```python
from build123d import *

# Parameters (mm, degrees)
ESQUISSE20_R        = 1.5
BOSS_EXTRU_18_DEPTH = 3


with BuildPart() as part:
    # Esquisse20 → Boss.-Extru.18 (new body)
    with BuildSketch(Plane.XY):
        with BuildLine():
            Line((110.974145272, 39.836071078), (121.886788051, 41.354939341))
            Line((121.886788051, 41.354939341), (126.749523122, 37.68045145))
            Line((126.749523122, 37.68045145), (136.453547574, 39.031099049))
            ThreePointArc((136.453547574, 39.031099049), (136.70394605, 39.25838517), (136.583626314, 39.574425576))
            Line((136.583626314, 39.574425576), (122.215724565, 49.579536305))
            Line((122.215724565, 49.579536305), (109.446142116, 47.334623838))
            ThreePointArc((109.446142116, 47.334623838), (109.157676293, 47.445546281), (109.120229419, 47.752326416))
            ThreePointArc((109.120229419, 47.752326416), (109.228042095, 48.009211598), (109.32429992, 48.270646104))
            ThreePointArc((109.32429992, 48.270646104), (109.335764075, 48.421294196), (109.272350858, 48.558425661))
            ThreePointArc((109.272350858, 48.558425661), (109.097464559, 48.765803687), (108.917279288, 48.968594544))
            ThreePointArc((108.917279288, 48.968594544), (108.79064668, 49.050998774), (108.639910127, 49.061234313))
            ThreePointArc((108.639910127, 49.061234313), (107.261509219, 48.631031321), (106.01862318, 47.895981682))
            ThreePointArc((106.01862318, 47.895981682), (105.838096498, 47.834835241), (105.657168579, 47.894784036))
            ThreePointArc((105.657168579, 47.894784036), (105.512617586, 48.000463717), (105.365584876, 48.10266238))
            ThreePointArc((105.365584876, 48.10266238), (105.21615426, 48.20132177), (105.064410914, 48.296385651))
            ThreePointArc((105.064410914, 48.296385651), (104.94165105, 48.44218958), (104.931503697, 48.632520348))
            ThreePointArc((104.931503697, 48.632520348), (105.15332497, 50.059355658), (105.041782665, 51.499016031))
            ThreePointArc((105.041782665, 51.499016031), (104.976386869, 51.635213184), (104.85290368, 51.722265908))
            ThreePointArc((104.85290368, 51.722265908), (104.597758689, 51.814417397), (104.340318239, 51.899946795))
            ThreePointArc((104.340318239, 51.899946795), (104.189449068, 51.907994647), (104.053789615, 51.841490608))
            ThreePointArc((104.053789615, 51.841490608), (103.075160908, 50.779723434), (102.366314843, 49.521708754))
            ThreePointArc((102.366314843, 49.521708754), (102.240547371, 49.378491042), (102.053884799, 49.339944262))
            ThreePointArc((102.053884799, 49.339944262), (101.875860127, 49.359190054), (101.697426734, 49.374180337))
            ThreePointArc((101.697426734, 49.374180337), (101.518686329, 49.384906567), (101.339740796, 49.39136263))
            ThreePointArc((101.339740796, 49.39136263), (101.160525671, 49.456252605), (101.056572421, 49.616010208))
            ThreePointArc((101.056572421, 49.616010208), (100.535257624, 50.96259647), (99.718828968, 52.153607774))
            ThreePointArc((99.718828968, 52.153607774), (99.59409597, 52.23886007), (99.44363003, 52.252508346))
            ThreePointArc((99.44363003, 52.252508346), (99.176592242, 52.204741381), (98.910877573, 52.150091787))
            ThreePointArc((98.910877573, 52.150091787), (98.776197112, 52.081626847), (98.691964599, 51.956202932))
            ThreePointArc((98.691964599, 51.956202932), (98.375330865, 50.547371233), (98.390459505, 49.10347553))
            ThreePointArc((98.390459505, 49.10347553), (98.353150535, 48.916561617), (98.210769396, 48.78984784))
            ThreePointArc((98.210769396, 48.78984784), (98.046972612, 48.717502849), (97.884949619, 48.641268118))
            ThreePointArc((97.884949619, 48.641268118), (97.724792772, 48.561187104), (97.566593363, 48.477305452))
            ThreePointArc((97.566593363, 48.477305452), (97.378943525, 48.443894256), (97.209038568, 48.530271774))
            ThreePointArc((97.209038568, 48.530271774), (96.08427358, 49.435792287), (94.781719971, 50.059024004))
            ThreePointArc((94.781719971, 50.059024004), (94.631071878, 50.070488159), (94.493940414, 50.007074943))
            ThreePointArc((94.493940414, 50.007074943), (94.286562388, 49.832188643), (94.083771531, 49.652003372))
            ThreePointArc((94.083771531, 49.652003372), (94.001367301, 49.525370764), (93.991131762, 49.374634211))
            ThreePointArc((93.991131762, 49.374634211), (94.421334754, 47.996233303), (95.156384393, 46.753347264))
            ThreePointArc((95.156384393, 46.753347264), (95.217530833, 46.572820582), (95.157582038, 46.391892663))
            ThreePointArc((95.157582038, 46.391892663), (95.051902358, 46.24734167), (94.949703695, 46.100308961))
            ThreePointArc((94.949703695, 46.100308961), (94.851044305, 45.950878344), (94.755980424, 45.799134999))
            ThreePointArc((94.755980424, 45.799134999), (94.610176495, 45.676375134), (94.419845727, 45.666227781))
            ThreePointArc((94.419845727, 45.666227781), (92.993010417, 45.888049055), (91.553350043, 45.77650675))
            ThreePointArc((91.553350043, 45.77650675), (91.417152891, 45.711110954), (91.330100167, 45.587627765))
            ThreePointArc((91.330100167, 45.587627765), (91.237948678, 45.332482774), (91.15241928, 45.075042323))
            ThreePointArc((91.15241928, 45.075042323), (91.144371427, 44.924173153), (91.210875467, 44.788513699))
            ThreePointArc((91.210875467, 44.788513699), (92.272642641, 43.809884992), (93.530657321, 43.101038928))
            ThreePointArc((93.530657321, 43.101038928), (93.673875032, 42.975271455), (93.712421813, 42.788608884))
            ThreePointArc((93.712421813, 42.788608884), (93.693176021, 42.610584211), (93.678185738, 42.432150818))
            ThreePointArc((93.678185738, 42.432150818), (93.667459507, 42.253410413), (93.661003444, 42.07446488))
            ThreePointArc((93.661003444, 42.07446488), (93.59611347, 41.895249755), (93.436355867, 41.791296505))
            ThreePointArc((93.436355867, 41.791296505), (92.089769605, 41.269981709), (90.8987583, 40.453553052))
            ThreePointArc((90.8987583, 40.453553052), (90.813506004, 40.328820055), (90.799857729, 40.178354115))
            ThreePointArc((90.799857729, 40.178354115), (90.847624694, 39.911316326), (90.902274287, 39.645601657))
            ThreePointArc((90.902274287, 39.645601657), (90.970739228, 39.510921196), (91.096163143, 39.426688683))
            ThreePointArc((91.096163143, 39.426688683), (92.504994842, 39.110054949), (93.948890545, 39.12518359))
            ThreePointArc((93.948890545, 39.12518359), (94.135804458, 39.08787462), (94.262518234, 38.945493481))
            ThreePointArc((94.262518234, 38.945493481), (94.334863226, 38.781696696), (94.411097956, 38.619673703))
            ThreePointArc((94.411097956, 38.619673703), (94.491178971, 38.459516856), (94.575060623, 38.301317448))
            ThreePointArc((94.575060623, 38.301317448), (94.608471819, 38.113667609), (94.522094301, 37.943762652))
            ThreePointArc((94.522094301, 37.943762652), (93.616573788, 36.818997664), (92.993342071, 35.516444055))
            ThreePointArc((92.993342071, 35.516444055), (92.981877915, 35.365795963), (93.045291132, 35.228664498))
            ThreePointArc((93.045291132, 35.228664498), (93.220177431, 35.021286472), (93.400362702, 34.818495616))
            ThreePointArc((93.400362702, 34.818495616), (93.526995311, 34.736091385), (93.677731863, 34.725855847))
            ThreePointArc((93.677731863, 34.725855847), (95.056132772, 35.156058839), (96.299018811, 35.891108478))
            ThreePointArc((96.299018811, 35.891108478), (96.479545492, 35.952254918), (96.660473412, 35.892306123))
            ThreePointArc((96.660473412, 35.892306123), (96.805024404, 35.786626442), (96.952057114, 35.684427779))
            ThreePointArc((96.952057114, 35.684427779), (97.101487731, 35.585768389), (97.253231076, 35.490704508))
            ThreePointArc((97.253231076, 35.490704508), (97.37599094, 35.344900579), (97.386138294, 35.154569811))
            ThreePointArc((97.386138294, 35.154569811), (97.16431702, 33.727734502), (97.275859325, 32.288074128))
            ThreePointArc((97.275859325, 32.288074128), (97.341255121, 32.151876975), (97.46473831, 32.064824252))
            ThreePointArc((97.46473831, 32.064824252), (97.719883301, 31.972672762), (97.977323751, 31.887143364))
            ThreePointArc((97.977323751, 31.887143364), (98.128192922, 31.879095512), (98.263852376, 31.945599551))
            ThreePointArc((98.263852376, 31.945599551), (99.242481083, 33.007366725), (99.951327147, 34.265381405))
            ThreePointArc((99.951327147, 34.265381405), (100.077094619, 34.408599117), (100.263757191, 34.447145897))
            ThreePointArc((100.263757191, 34.447145897), (100.441781863, 34.427900105), (100.620215257, 34.412909822))
            ThreePointArc((100.620215257, 34.412909822), (100.798955662, 34.402183592), (100.977901194, 34.395727529))
            ThreePointArc((100.977901194, 34.395727529), (101.15711632, 34.330837554), (101.26106957, 34.171079951))
            ThreePointArc((101.26106957, 34.171079951), (101.782384366, 32.824493689), (102.598813023, 31.633482385))
            ThreePointArc((102.598813023, 31.633482385), (102.72354602, 31.548230089), (102.87401196, 31.534581813))
            ThreePointArc((102.87401196, 31.534581813), (103.141049749, 31.582348778), (103.406764418, 31.636998372))
            ThreePointArc((103.406764418, 31.636998372), (103.541444878, 31.705463312), (103.625677392, 31.830887227))
            ThreePointArc((103.625677392, 31.830887227), (103.942311126, 33.239718926), (103.927182485, 34.683614629))
            ThreePointArc((103.927182485, 34.683614629), (103.964491455, 34.870528542), (104.106872594, 34.997242319))
            ThreePointArc((104.106872594, 34.997242319), (104.270669379, 35.06958731), (104.432692372, 35.145822041))
            ThreePointArc((104.432692372, 35.145822041), (104.592849218, 35.225903055), (104.751048627, 35.309784707))
            ThreePointArc((104.751048627, 35.309784707), (104.938698466, 35.343195904), (105.108603422, 35.256818386))
            ThreePointArc((105.108603422, 35.256818386), (106.233368411, 34.351297873), (107.53592202, 33.728066155))
            ThreePointArc((107.53592202, 33.728066155), (107.686570112, 33.716602), (107.823701576, 33.780015217))
            ThreePointArc((107.823701576, 33.780015217), (108.031079603, 33.954901516), (108.233870459, 34.135086787))
            ThreePointArc((108.233870459, 34.135086787), (108.316274689, 34.261719395), (108.326510228, 34.412455948))
            ThreePointArc((108.326510228, 34.412455948), (107.896307236, 35.790856856), (107.161257597, 37.033742895))
            ThreePointArc((107.161257597, 37.033742895), (107.100111157, 37.214269577), (107.160059952, 37.395197496))
            ThreePointArc((107.160059952, 37.395197496), (107.265739633, 37.539748489), (107.367938296, 37.686781199))
            ThreePointArc((107.367938296, 37.686781199), (107.466597686, 37.836211815), (107.561661567, 37.987955161))
            ThreePointArc((107.561661567, 37.987955161), (107.707465496, 38.110715025), (107.897796264, 38.120862378))
            ThreePointArc((107.897796264, 38.120862378), (109.324631573, 37.899041104), (110.764291947, 38.010583409))
            ThreePointArc((110.764291947, 38.010583409), (110.9004891, 38.075979206), (110.987541823, 38.199462394))
            ThreePointArc((110.987541823, 38.199462394), (111.079693313, 38.454607385), (111.165222711, 38.712047836))
            ThreePointArc((111.165222711, 38.712047836), (111.173270563, 38.862917007), (111.106766523, 38.99857646))
            ThreePointArc((111.106766523, 38.99857646), (110.95766042, 39.16577253), (110.802658091, 39.327517495))
            ThreePointArc((110.802658091, 39.327517495), (110.731228871, 39.634793859), (110.974145272, 39.836071078))
        make_face()
        with Locations((101.158820995, 41.89354508)):
            Circle(ESQUISSE20_R, mode=Mode.SUBTRACT)
    extrude(amount=BOSS_EXTRU_18_DEPTH)


solid = part.part
```
The model under review builds one solid part; all positions refer to its coordinate system, in mm. A direction names the side the tool comes from. Give positions to 0.01 mm unless a question says otherwise; leave off trailing zeros. Write each loop counter-clockwise with the first axis right and the second up, starting at its lowest first coordinate (ties: lowest second). Pieces come first, ordered by that corner, then holes. Notation, with made-up numbers: (76, 73.25) -> (125, 73.25) arc R12 ccw to (125, 84.25) -> close; hole circle Ø3 at (3.5, 43). An arc over 180 degrees is marked (long way). Answer in a Markdown table with one row per item.
1) Clearance check with a flat-ended pin moving along its axis: P1, Ø2.5, axis at x = 101.16, y = 41.89, coming from the -Z side. State where the tip first meets the part, or that it passes through.
Worked answers:
| item | result |
|---|---|
| P1 | through |
2) Add section B-B on x = 130. State the section outline as (y, z) points, plus the area to 3 significant figures.
Worked answers:
| item | result |
|---|---|
| outline | (38.13, 0) -> (44.16, 0) -> (44.16, 3) -> (38.13, 3) -> close |
| area | 18.1 mm² |
3) Add section A-A on x = 116. State the section outline as (y, z) points.
Worked answers:
| item | result |
|---|---|
| outline | (40.54, 0) -> (48.49, 0) -> (48.49, 3) -> (40.54, 3) -> close |
4) Tool access review of faces 1 (the cylindrical face through (107.905, 35.772, 1.479)), 2 (the flat face through (124.284, 39.543, 1.479)), 3 (the cylindrical face through (98.377, 50.568, 1.479)): name each direction out of +Z, -Z, +X, -X, +Y, -Y from which nothing blocks a thin tool from reaching the whole face with its end or side.
Worked answers:
| item | result |
|---|---|
| face 1 | +Z, -Z, +X |
| face 2 | +Z, -Z, -Y |
| face 3 | +Z, -Z |
5) Mouldability with a two-part tool opening along X and no side actions: class faces 4 (the cylindrical face through (100.545, 50.945, 1.479)), 5 (the flat face through (108, 42, 3)), 6 (the flat face through (116.354, 40.585, 1.479)), 7 (the cylindrical face through (92.11, 41.28, 1.48)) as +X half, -X half, draft (parallel to the pull), parting line (faces both ways), or undercut.
Worked answers:
| item | result |
|---|---|
| face 4 | undercut |
| face 5 | draft |
| face 6 | undercut |
| face 7 | -X half |
6) For L1, parallel to X at y = 50.5, z = 1.35; L2, parallel to X at y = 32.75, z = 1.6; L3, parallel to Y at x = 127.5, z = 1.8, list the stretches that pass through material, from the lowest coordinate up. Write a range as [from, to].
Worked answers:
| item | result |
|---|---|
| L1 | [98.37, 100.76], [102.88, 105.15] |
| L2 | [97.2, 99.04], [101.82, 103.87] |
| L3 | [37.78, 45.9] |
